Geometry check sheet. Reference: the model listing, model coordinates, mm. A direction names the side the tool comes from. Coordinates: 2 decimals unless noted, no trailing zeros. Write each loop counter-clockwise with the first axis right and the second up, starting at its lowest first coordinate (ties: lowest second). Pieces come first, ordered by that corner, then holes. Notation, with made-up numbers: M 0.5,11.5 L 54.5,11.5 A22 ccw 54.5,27.5 Z; hole C -4.5,68.5 d9. An arc over 180 degrees is marked long. Put each result on its own line as item: value. Start each with the question number.
1) Cross-section at D-D on z = 2.25. Record the cut outline in (x, y).
2) Cross-section at B-B on z = 11. Record the cut outline in (x, y), plus the area to 3 significant figures.
3) Gauge pin test, flat ends, axial feed: pin 1 (10 mm diameter, centred on x = -3.5, y = -1, fed in from -Z); pin 2 (1.5 mm diameter, centred on y = 1, z = 6, fed in from +X); pin 3 (3.5 mm diameter, centred on x = -1.5, y = 2, fed in from +Z); pin 4 (4.5 mm diameter, centred on x = 0, z = 9.5, fed in from -Y). Record the tip position at first contact, or that the pin passes through.
4) Scan lines: line 1 along Y through (x, z) = (9.25, 0.7); line 2 along X through (y, z) = (-0.75, 2.5); line 3 along Y through (x, z) = (-0.25, 11). Record each from-to range of solid material in increasing order.
5) Cross-section at C-C on y = 3.5. Record the cut outline in (x, z), plus the area to 4 significant figures.
6) Cross-section at A-A on x = 9.25. Record the cut outline in (y, z).
7) Set-up check for faces 4 (the flat face through (1, -7.5, 7)), 5 (the flat face through (7, 0, 3)), 6 (the flat face through (1, 7.5, 7)): record each of +Z, -Z, +X, -X, +Y, -Y from which the full face is reachable in a straight line by a thin tool's end or side.
8) Mould release check, pull along X, two halves, no side actions. Record for faces 1 (the flat face through (-9.21, 5.98, 8.07)), 2 (the cylindrical face through (-7.581, 0.526, 1.479)), 3 (the flat face through (0, -9, 3)): released by +X, released by -X, zero draft, split by the parting line, or undercut.
from build123d import *

# Parameters (mm, degrees)
ESQUISSE1_W               = 24
ESQUISSE1_H               = 20
ESQUISSE1_R               = 1.75
ESQUISSE1_W_2             = 13
ESQUISSE1_H_2             = 15
BOSS_EXTRU_1_DEPTH        = 3
ESQUISSE1_3_W             = 13
ESQUISSE1_3_H             = 15
ESQUISSE1_3_W_2           = 7
ESQUISSE1_3_H_2           = 9
BOSS_EXTRU_2_DEPTH        = 13
NERVURE2_REACH            = 26.885
ESQUISSE5_WALL_W          = 63.182180764
ESQUISSE5_WALL_H          = 3
SYM_TRIE5_COPY_1_REACH    = 26.885
SYM_TRIE5_COPY_1_SKETCH_W = 63.182180764
SYM_TRIE5_COPY_1_SKETCH_H = 3
ESQUISSE1_4_W             = 7
ESQUISSE1_4_H             = 9
BOSS_EXTRU_3_DEPTH        = 7.5


with BuildPart() as part:
    # Esquisse1 → Boss.-Extru.1 (new body)
    with BuildSketch(Plane.XY):
        Rectangle(ESQUISSE1_W, ESQUISSE1_H)
        with Locations((-9.25, 0)):
            Circle(ESQUISSE1_R, mode=Mode.SUBTRACT)
        with Locations((9.25, 0)):
            Circle(ESQUISSE1_R, mode=Mode.SUBTRACT)
        Rectangle(ESQUISSE1_W_2, ESQUISSE1_H_2, mode=Mode.SUBTRACT)
    extrude(amount=BOSS_EXTRU_1_DEPTH)

    # Esquisse1<3> → Boss.-Extru.2 (add)
    with BuildSketch(Plane.XY):
        Rectangle(ESQUISSE1_3_W, ESQUISSE1_3_H)
        Rectangle(ESQUISSE1_3_W_2, ESQUISSE1_3_H_2, mode=Mode.SUBTRACT)
    extrude(amount=BOSS_EXTRU_2_DEPTH)

    # Esquisse5 wall → Nervure2 (add, up to next)
    with BuildSketch(Plane(origin=(-9.25, -7.5, 8), x_dir=(-0.481918749772, 0, -0.876215908677), z_dir=(0.876215908677, 0, -0.481918749772)), mode=Mode.PRIVATE) as nervure2_sk1:
        with Locations((0, 1.5)):
            Rectangle(ESQUISSE5_WALL_W, ESQUISSE5_WALL_H)
    nervure2_tool1 = extrude(nervure2_sk1.sketch, amount=NERVURE2_REACH, mode=Mode.PRIVATE) - part.part
    nervure2 = nervure2_tool1.solids().sort_by_distance((-9.25, -7.5, 8))[0]
    add(nervure2)

    # Symétrie4: Nervure2 across plane
    add(nervure2.mirror(Plane.ZX))

    # Symétrie5: Nervure2 across plane
    add(nervure2.mirror(Plane(origin=(0, 0, 0), x_dir=(0, 0, 1), z_dir=(1, 0, 0))))

    # Symétrie5 copy 1 sketch → Symétrie5 copy 1 (add, up to next)
    with BuildSketch(Plane(origin=(9.25, 7.5, 8), x_dir=(0.481918749772, 0, -0.876215908677), z_dir=(-0.876215908677, 0, -0.481918749772)), mode=Mode.PRIVATE) as sym_trie5_copy_1_sk1:
        with Locations((0, 1.5)):
            Rectangle(SYM_TRIE5_COPY_1_SKETCH_W, SYM_TRIE5_COPY_1_SKETCH_H)
    sym_trie5_copy_1_tool1 = extrude(sym_trie5_copy_1_sk1.sketch, amount=SYM_TRIE5_COPY_1_REACH, mode=Mode.PRIVATE) - part.part
    add(sym_trie5_copy_1_tool1.solids().sort_by_distance((9.25, 7.5, 8))[0])

    # Esquisse1<4> → Boss.-Extru.3 (add)
    with BuildSketch(Plane.XY):
        Rectangle(ESQUISSE1_4_W, ESQUISSE1_4_H)
    extrude(amount=BOSS_EXTRU_3_DEPTH)


solid = part.part
Answer key:
1. outline: M -12,-10 L 12,-10 L 12,10 L -12,10 Z; hole C -9.25,0 d3.5; hole C 9.25,0 d3.5
2. outline: M -7.6,-7.5 L 7.6,-7.5 L 7.6,-4.5 L 6.5,-4.5 L 6.5,4.5 L 7.6,4.5 L 7.6,7.5 L -7.6,7.5 L -7.6,4.5 L -6.5,4.5 L -6.5,-4.5 L -7.6,-4.5 Z; hole M -3.5,-4.5 L 3.5,-4.5 L 3.5,4.5 L -3.5,4.5 Z
2. area: 145 mm²
3. pin 1: stops at z = 0
3. pin 2: stops at x = 6.5
3. pin 3: stops at z = 7.5
3. pin 4: stops at y = -7.5
4. line 1: y = -10 to -1.75, 1.75 to 10
4. line 2: x = -12 to -10.83, -7.67 to 7.67, 10.83 to 12
4. line 3: y = -7.5 to -4.5, 4.5 to 7.5
5. outline: M -12,0 L 12,0 L 12,3 L 6.5,3 L 6.5,13 L 3.5,13 L 3.5,7.5 L -3.5,7.5 L -3.5,13 L -6.5,13 L -6.5,3 L -12,3 Z
5. area: 163.5 mm²
6. outline: M -10,0 L -1.75,0 L -1.75,3 L -4.5,3 L -4.5,8 L -7.5,8 L -7.5,3 L -10,3 Z; M 1.75,0 L 10,0 L 10,3 L 7.5,3 L 7.5,8 L 4.5,8 L 4.5,3 L 1.75,3 Z
7. face 4: +Z, +X, -X, -Y
7. face 5: +Z, +X
7. face 6: +Z, +X, -X, +Y
8. face 1: released by -X
8. face 2: undercut
8. face 3: zero draft
